Geometry check sheet. Reference: the model listing, model coordinates, mm. Face numbers are marked on the shaded views. A direction names the side the tool comes from. Round coordinates to 2 decimals unless told otherwise and drop trailing zeros. Loops run counter-clockwise (first coordinate to the right, second up) from the corner with the lowest first, then second, coordinate; pieces in that order, holes last. Notation, with made-up numbers: M 57.5,84.5 L 106.5,84.5 A23 ccw 106.5,108.5 Z; hole C -25.5,50.25 d10. An arc over 180 degrees is marked long. Answer in a Markdown table with one row per item. Add a question column.
Autodesk Inventor part; units mm, degrees
ref_plane "Work Plane1" through (0, 56, 0) normal (0, 1, 0) x (1, 0, 0)
ref_plane "YZ Plane" through (0, 0, 0) normal (1, 0, 0) x (0, 1, 0)
ref_plane "XZ Plane" through (0, 0, 0) normal (0, 1, 0) x (-1, 0, 0)
sketch "Sketch1" plane through (0, 0, 0) normal (0, 1, 0) x (-1, 0, 0)
  line L0 (0, 0) -> (-20, 0)
  line L1 (-20, 0) -> (-20, -41)
  line L2 (-20, -41) -> (0, -41)
  line L3 (0, -41) -> (0, 0)
  dimension "d0" = 20
  dimension "d1" = 41
extrude "Extrusion1" add sketch "Sketch1" along normal blind 24
sketch "Sketch2" plane through (0, 24, 0) normal (0, 1, 0) x (1, 0, 0)
  line L0 (0, 41) -> (0, 0)
  line L1 (0, 0) -> (0, -5)
  line L2 (0, -5) -> (20, -5)
  line L3 (20, -5) -> (20, 46)
  line L4 (20, 46) -> (0, 46)
  line L5 (0, 46) -> (0, -5)
  line L6 (0, -4) -> (5, -4)
  circle A0 centre (5, -4) radius 2
  line L7 (5, -4) -> (15, -4)
  circle A1 centre (15, -4) radius 2
  line L8 (0, 0) -> (0, 20.5)
  line L9 (0, 20.5) -> (20, 20.5)
  line L10 (20, 0) -> (20, 41)
  line L11 (0, 45) -> (5, 45)
  circle A2 centre (5, 45) radius 2
  circle A3 centre (15, 45) radius 2
  line L12 (0, 0) -> (20, 0)
  point P0 (3.2679, -5)
  point P1 (6.7321, -5)
  point P2 (13.2679, -5)
  point P3 (16.7321, -5)
  point P4 (16.7321, 46)
  point P5 (13.2679, 46)
  point P6 (6.7321, 46)
  point P7 (3.2679, 46)
  dimension "d4" = 5
  dimension "d5" = 20
  dimension "d6" = 51
  dimension "d7" = 5
  dimension "d8" = 4
  dimension "d9" = 10
  dimension "d10" = 4
  dimension "d11" = 20.5
  dimension "d29" = 4
extrude "Extrusion2" add sketch "Sketch2" along normal blind 2 contours L5 L11 A2 L4 A3 L3 L9 L0 | L9 L3 L12 L0 | L5 L4 A2 L11 | L12 L3 L2 A1 L7 A0 L6 L1 | L6 A0 L2 L1 | L7 A1 L2 A0
sketch "Sketch3" plane through (0, 26, 0) normal (0, 1, 0) x (1, 0, 0)
  line L0 (0, 46) -> (0, -5)
  line L1 (0, -5) -> (0, 10)
  line L2 (0, 10) -> (10.5, 10)
  circle A0 centre (10.5, 10) radius 2.5
  circle A1 centre (10.5, 10) radius 4
  circle A2 centre (10.5, 10) radius 7.5
  circle A3 centre (10.5, 10) radius 1.5
  point P0 (0, 0)
  dimension "d14" = 15
  dimension "d15" = 10.5
  dimension "d16" = 5
  dimension "d17" = 8
  dimension "d18" = 15
  dimension "d19" = 3
extrude "Extrusion3" add sketch "Sketch3" along normal blind 13 contours A0
extrude "Extrusion4" add sketch "Sketch3" along normal blind 4 contours A1
extrude "Extrusion5" add sketch "Sketch3" along normal blind 2 contours A2
sketch "Sketch4" plane through (0, 0, 0) normal (0, 0, 1) x (1, 0, 0)
  line L0 (20, 0) -> (0, 0)
  line L1 (7.8843, 0) -> (13.1114, 0)
  line L2 (13.1114, 0) -> (13.1114, 2.57)
  line L3 (13.1114, 2.57) -> (7.8843, 2.57)
  line L4 (7.8843, 2.57) -> (7.8843, 0)
extrude "Extrusion6" add sketch "Sketch4" along normal blind 3
ref_plane "Work Plane1" through (0, 56, 0) normal (0, 1, 0) x (1, 0, 0)
sketch "Sketch5" plane through (0, 56, 0) normal (0, 1, 0) x (1, 0, 0)
  circle A0 centre (10.5, 10) radius 7.5
  line L0 (0, 46) -> (0, -5)
  line L1 (0, -5) -> (3.2679, -5)
  arc A1 (6.7321, -5) -> (3.2679, -5) centre (5, -4) ccw
  line L2 (6.7321, -5) -> (13.2679, -5)
  arc A2 (16.7321, -5) -> (13.2679, -5) centre (15, -4) ccw
  line L3 (16.7321, -5) -> (20, -5)
  line L4 (20, -5) -> (20, 46)
  line L5 (20, 46) -> (16.7321, 46)
  arc A3 (13.2679, 46) -> (16.7321, 46) centre (15, 45) ccw
  line L6 (13.2679, 46) -> (6.7321, 46)
  arc A4 (3.2679, 46) -> (6.7321, 46) centre (5, 45) ccw
  line L7 (3.2679, 46) -> (0, 46)
  circle A5 centre (10.5, 10) radius 2.5
  circle A6 centre (10.5, 10) radius 4
  circle A7 centre (10.5, 10) radius 1.5
  point P0 (0, 0)
properties part number "servo"
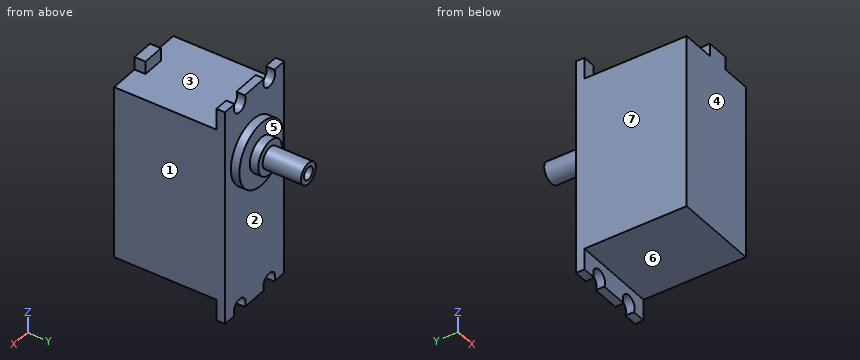
1) Set-up check for the marked faces 5, 6 and 7: record each of +Z, -Z, +X, -X, +Y, -Y from which the full face is reachable in a straight line by a thin tool's end or side.
2) Cross-section at C-C, the plane y = 34. Record the boundary of the cut face in (x, z), plus the area to 3 significant figures.
3) Draft check along Y on the marked faces 1, 2, 3 and 4. Enter one of: +Y half, -Y half, draft (parallel to the pull), parting line (faces both ways), or undercut.
4) Cross-section at A-A, the plane z = -45. Record the boundary of the cut face in (x, y).
5) Go/stop test with flat-tipped pins: pin 1 (10 mm diameter, centred on x = 13.5, y = 12, fed in from -Z); pin 2 (5 mm diameter, centred on x = 5.5, y = 17, fed in from +Z); pin 3 (6.5 mm diameter, centred on x = 11.5, z = -9, fed in from +Y); pin 4 (1.5 mm diameter, centred on x = 3.5, z = -10, fed in from +Y). Record where each tip stops, or that it passes through.
6) Cross-section at B-B, the plane x = 10.5. Record the boundary of the cut face in (y, z), plus the area to 3 significant figures.
7) Cross-section at D-D, the plane z = -10. Record the boundary of the cut face in (x, y), plus the area to 3 significant figures.
8) Thickness scan on L1, parallel to X at y = 25.2, z = 4; L2, parallel to X at y = 35, z = -10; L3, parallel to Y at x = 5.25, z = -3.5. Record the ranges inside material, lowest first. Write a range as [from, to].
Worked answers:
| question | item | result |
|---|---|---|
| 1 | face 5 | +Y |
| 1 | face 6 | -Z, +X, -X, -Y |
| 1 | face 7 | +Z, -Z, -X, +Y, -Y |
| 2 | outline | C 10.5,-10 d5; hole C 10.5,-10 d3 |
| 2 | area | 12.6 mm2 |
| 3 | face 1 | draft |
| 3 | face 2 | +Y half |
| 3 | face 3 | undercut |
| 3 | face 4 | -Y half |
| 4 | outline | M 0,24 L 3,24 L 3,26 L 0,26 Z; M 7,24 L 13,24 L 13,26 L 7,26 Z; M 17,24 L 20,24 L 20,26 L 17,26 Z |
| 5 | pin 1 | stops at z = -41 |
| 5 | pin 2 | stops at z = 0 |
| 5 | pin 3 | stops at y = 39 |
| 5 | pin 4 | stops at y = 28 |
| 6 | outline | M 0,-41 L 24,-41 L 24,-46 L 26,-46 L 26,-17.5 L 28,-17.5 L 28,-14 L 30,-14 L 30,-12.5 L 39,-12.5 L 39,-11.5 L 26,-11.5 L 26,-8.5 L 39,-8.5 L 39,-7.5 L 30,-7.5 L 30,-6 L 28,-6 L 28,-2.5 L 26,-2.5 L 26,5 L 24,5 L 24,0 L 2.57,0 L 2.57,3 L 0,3 Z |
| 6 | area | 1,150 mm2 |
| 7 | outline | M 0,0 L 20,0 L 20,26 L 18,26 L 18,28 L 14.5,28 L 14.5,30 L 13,30 L 13,39 L 12,39 L 12,26 L 9,26 L 9,39 L 8,39 L 8,30 L 6.5,30 L 6.5,28 L 3,28 L 3,26 L 0,26 Z |
| 7 | area | 572 mm2 |
| 8 | L1 | x = [0, 3], [7, 13], [17, 20] |
| 8 | L2 | x = [8, 9], [12, 13] |
| 8 | L3 | y = [0, 26] |
